Read the model definition and answer for the solid it produces. Units are mm, in the model's axes. A direction names the side the tool comes from. Coordinates: 2 decimals unless noted, no trailing zeros. Order: outer loops, then holes, each group sorted by start corner. A loop starts at its lowest first (then second) coordinate and runs counter-clockwise, first axis right, second up.
```python
from build123d import *

# Parameters (mm, degrees)
SKETCH_1_W          = 30
SKETCH_1_H          = 40
SKETCH_1_W_2        = 27
SKETCH_1_H_2        = 37
EXTRUDE_1_DEPTH     = 100
SKETCH_3_R          = 1.525
CUT_EXTRUDE_2_DEPTH = 50
SKETCH_5_R          = 3.15
CUT_EXTRUDE_4_DEPTH = 3
SKETCH_6_R          = 2.525
CUT_EXTRUDE_5_DEPTH = 50
SKETCH_7_R          = 2.025
CUT_EXTRUDE_6_DEPTH = 10
SKETCH_8_R          = 3.5
CUT_EXTRUDE_7_DEPTH = 5


with BuildPart() as part:
    # Sketch 1 → Extrude 1 (new, symmetric)
    with BuildSketch(Plane.XY):
        Rectangle(SKETCH_1_W, SKETCH_1_H)
        Rectangle(SKETCH_1_W_2, SKETCH_1_H_2, mode=Mode.SUBTRACT)
    extrude(amount=EXTRUDE_1_DEPTH, both=True)

    # Sketch 3 → Cut-Extrude 2 (cut)
    with BuildSketch(Plane(origin=(0, 20, 0), x_dir=(1, 0, 0), z_dir=(0, 1, 0))):
        with Locations(Location((-7.5, 10, 0), (0, 0, 270))):
            Circle(SKETCH_3_R)
        with Locations(Location((-7.5, -10, 0), (0, 0, 270))):
            Circle(SKETCH_3_R)
    extrude(amount=-CUT_EXTRUDE_2_DEPTH, mode=Mode.SUBTRACT)

    # Sketch 5 → Cut-Extrude 4 (cut)
    with BuildSketch(Plane.XZ.offset(20)):
        with Locations(Location((-7.5, 10, 0), (0, 0, 270))):
            Circle(SKETCH_5_R)
        with Locations(Location((-7.5, -10, 0), (0, 0, 270))):
            Circle(SKETCH_5_R)
    extrude(amount=-CUT_EXTRUDE_4_DEPTH, mode=Mode.SUBTRACT)

    # Sketch 6 → Cut-Extrude 5 (cut)
    with BuildSketch(Plane(origin=(0, 20, 0), x_dir=(1, 0, 0), z_dir=(0, 1, 0))):
        with Locations(Location((5, 45, 0), (0, 0, 270))):
            Circle(SKETCH_6_R)
        with Locations(Location((5, -45, 0), (0, 0, 270))):
            Circle(SKETCH_6_R)
    extrude(amount=-CUT_EXTRUDE_5_DEPTH, mode=Mode.SUBTRACT)

    # Sketch 7 → Cut-Extrude 6 (cut)
    with BuildSketch(Plane.XZ.offset(-18.5)):
        with Locations(Location((-10, 94, 0), (0, 0, 270))):
            Circle(SKETCH_7_R)
        with Locations(Location((10, 94, 0), (0, 0, 270))):
            Circle(SKETCH_7_R)
        with Locations(Location((10, 66, 0), (0, 0, 270))):
            Circle(SKETCH_7_R)
        with Locations(Location((-10, 66, 0), (0, 0, 270))):
            Circle(SKETCH_7_R)
        with Locations(Location((10, -66, 0), (0, 0, 270))):
            Circle(SKETCH_7_R)
        with Locations(Location((-10, -66, 0), (0, 0, 270))):
            Circle(SKETCH_7_R)
        with Locations(Location((10, -94, 0), (0, 0, 270))):
            Circle(SKETCH_7_R)
        with Locations(Location((-10, -94, 0), (0, 0, 270))):
            Circle(SKETCH_7_R)
    extrude(amount=-CUT_EXTRUDE_6_DEPTH, mode=Mode.SUBTRACT)

    # Sketch 8 → Cut-Extrude 7 (cut, symmetric)
    with BuildSketch(Plane(origin=(0, -18.5, 0), x_dir=(1, 0, 0), z_dir=(0, 1, 0))):
        with Locations(Location((-10, 94, 0), (0, 0, 180))):
            Circle(SKETCH_8_R)
        with Locations((10, 94)):
            Circle(SKETCH_8_R)
        with Locations((10, 66)):
            Circle(SKETCH_8_R)
        with Locations(Location((-10, 66, 0), (0, 0, 180))):
            Circle(SKETCH_8_R)
        with Locations((10, -66)):
            Circle(SKETCH_8_R)
        with Locations(Location((-10, -66, 0), (0, 0, 180))):
            Circle(SKETCH_8_R)
        with Locations(Location((-10, -94, 0), (0, 0, 180))):
            Circle(SKETCH_8_R)
        with Locations((10, -94)):
            Circle(SKETCH_8_R)
    extrude(amount=CUT_EXTRUDE_7_DEPTH, both=True, mode=Mode.SUBTRACT)


solid = part.part
```
1) A cutting plane is placed at D-D, the plane x = 10. State how many separate pieces and enclosed holes the cut face has, and give its area (3 significant figures).
A:
separate pieces: 10
enclosed holes: 0
area: 534 mm2
2) A cutting plane is placed at A-A, the plane z = -45. Determine the outline of the cut face in (x, y) (3 decimals).
A:
outline: (-15, -20) - (2.475, -20) - (2.475, -18.5) - (-13.5, -18.5) - (-13.5, 18.5) - (2.475, 18.5) - (2.475, 20) - (-15, 20) - close; (7.525, -20) - (15, -20) - (15, 20) - (7.525, 20) - (7.525, 18.5) - (13.5, 18.5) - (13.5, -18.5) - (7.525, -18.5) - close
3) A cutting plane is placed at C-C, the plane y = 0.5. Determine the outline of the cut face in (x, z).
A:
outline: (-15, -100) - (-13.5, -100) - (-13.5, 100) - (-15, 100) - close; (13.5, -100) - (15, -100) - (15, 100) - (13.5, 100) - close
4) Which of the six approach directions +Z, -Z, +X, -X, +Y, -Y give full straight-line access (tool end or side, diameter ignored) to faces 1 (the flat face through (13.5, 0, 1)), 2 (the cylindrical face through (-5.37, -19.26, 12.32)), 3 (the cylindrical face through (5.111, -19.24, -47.523))?
A:
face 1: +Z, -Z
face 2: -Y
face 3: +Y, -Y
5) Straight lines are drawn through the part: line 1 (Z direction, x = 10, y = -19.35); line 2 (X direction, y = 19.6, z = -94) (3 decimals); line 3 (Y direction, x = 4.75, z = -80.5). For each, find the intervals that lie inside material, in ascending order.
A:
line 1: z = -100 to -97.5, -90.5 to -69.5, -62.5 to 62.5, 69.5 to 90.5, 97.5 to 100
line 2: x = -15 to -12.025, -7.975 to 7.975, 12.025 to 15
line 3: y = -20 to -18.5, 18.5 to 20
6) Determine the mould class of faces 4 (the cylindrical face through (-9.241, -19.24, -97.417)), 5 (the cylindrical face through (5.111, 19.26, 42.477)), 6 (the flat face through (0, 18.5, 1)) for opening direction Z: pulls with the +Z half, pulls with the -Z half, needs draft (parallel to the pull), parting line crosses it, or undercut.
A:
face 4: undercut
face 5: undercut
face 6: needs draft
7) A cutting plane is placed at B-B, the plane x = -0.75. Determine the outline of the cut face in (y, z).
A:
outline: (-20, -100) - (-18.5, -100) - (-18.5, 100) - (-20, 100) - close; (18.5, -100) - (20, -100) - (20, 100) - (18.5, 100) - close
8) Flat-ended cylindrical pins translate along their axes: pin 1 Ø6.5 at (x, z) = (10, -94) entering from +Y; pin 2 Ø3.5 at (x, z) = (-7.5, 10) entering from -Y; pin 3 Ø3.5 at (x, z) = (-10, -66) entering from -Y. Find the tip coordinate at first contact, or state that the pin passes through.
A:
pin 1: stops at y = 20
pin 2: stops at y = 18.5
pin 3: passes through
